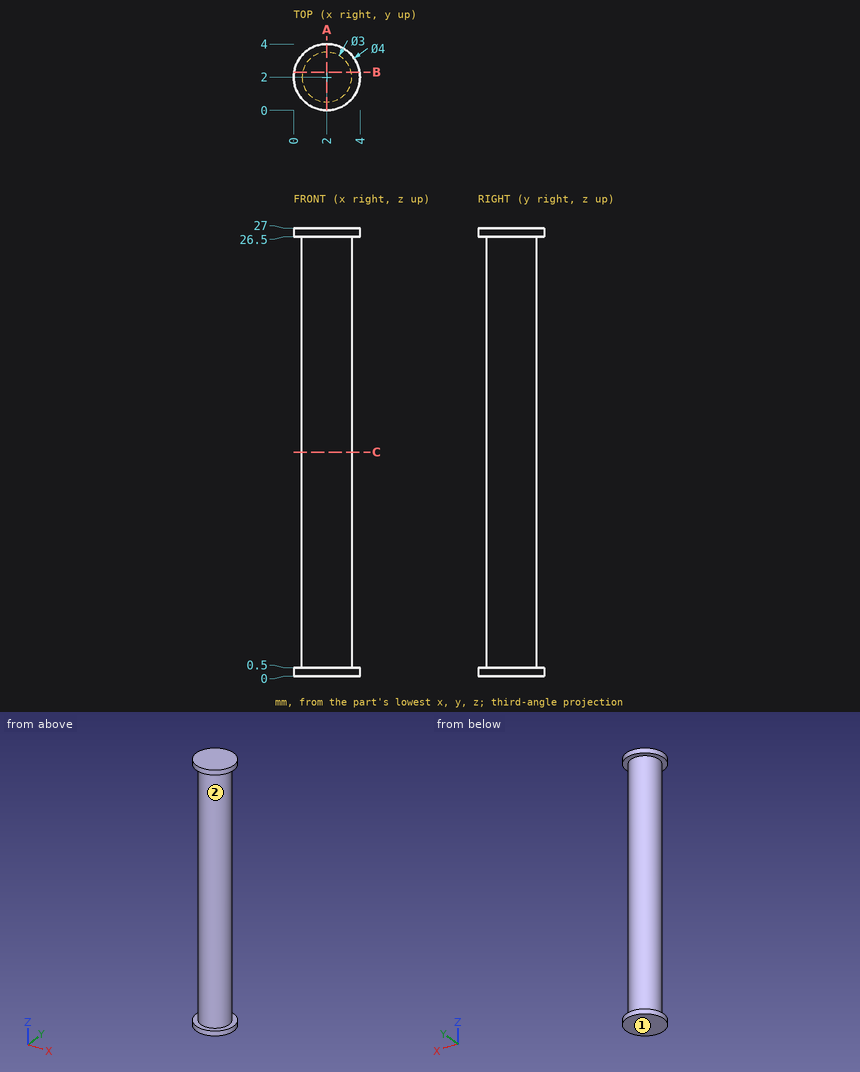
Check sheet for the drawn part. Datum: minimum x, y, z corner. Units: mm. A direction names the side the tool comes from. Give positions to 0.01 mm unless a question says otherwise; leave off trailing zeros. Loops run counter-clockwise (first coordinate to the right, second up) from the corner with the lowest first, then second, coordinate; pieces in that order, holes last.
1) Sectioned sample at B-B, the plane y = 2.3. Enter the section's corners in (x, z).
2) Sectioned sample at A-A, the plane x = 2. Enter the section's corners in (y, z).
3) Sectioned sample at C-C, the plane z = 13.5. Enter the section's corners in (x, y).
4) Thickness scan on line 1 along Z through (x, y) = (2.7, 3.7); line 2 along Y through (x, z) = (2, 2.25). Record the ranges inside material, lowest first.
5) Set-up check for the marked faces 1 and 2: record each of +Z, -Z, +X, -X, +Y, -Y from which the full face is reachable in a straight line by a thin tool's end or side.
6) Depth check by flat-ended pin: pin 1 Ø1.5 at (x, z) = (1, 10.5) entering from +Y. Enter the tip coordinate at first touch or a pass-through.
Answers:
1. outline: (0.02, 0) - (3.98, 0) - (3.98, 0.5) - (3.47, 0.5) - (3.47, 26.5) - (3.98, 26.5) - (3.98, 27) - (0.02, 27) - (0.02, 26.5) - (0.53, 26.5) - (0.53, 0.5) - (0.02, 0.5) - close
2. outline: (0, 0) - (4, 0) - (4, 0.5) - (3.5, 0.5) - (3.5, 26.5) - (4, 26.5) - (4, 27) - (0, 27) - (0, 26.5) - (0.5, 26.5) - (0.5, 0.5) - (0, 0.5) - close
3. outline: circle Ø3 at (2, 2)
4. line 1: z = 0 to 0.5, 26.5 to 27
4. line 2: y = 0.5 to 3.5
5. face 1: -Z, +X, -X, +Y, -Y
5. face 2: none
6. pin 1: stops at y = 3.48
